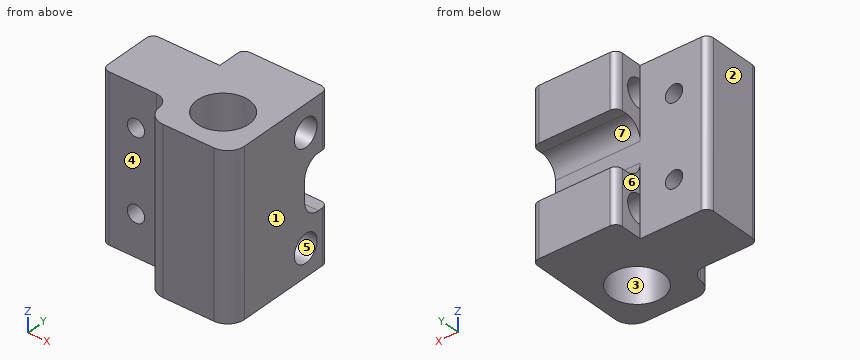
from build123d import *

# Parameters (mm, degrees)
SKETCH_1_W          = 25
SKETCH_1_H          = 48
EXTRUDE_1_DEPTH     = 25
SKETCH_2_R          = 7.65
CUT_EXTRUDE_1_DEPTH = 57.57461336
SKETCH_3_W          = 25
SKETCH_3_H          = 48
EXTRUDE_2_DEPTH     = 10
SKETCH_4_R          = 4.1
CUT_EXTRUDE_2_DEPTH = 53.240311871
FILLET_1_R          = 5
SKETCH_6_W          = 48
SKETCH_6_H          = 18
EXTRUDE_3_DEPTH     = 20
SKETCH_7_R          = 2.55
CUT_EXTRUDE_3_DEPTH = 54.919821703
FILLET_3_R          = 4
SKETCH_8_W          = 25
SKETCH_8_H          = 16
CUT_EXTRUDE_4_DEPTH = 8.406306785
FILLET_4_R          = 5
FILLET_5_R          = 2
FILLET_6_R          = 2


with BuildPart() as part:
    # 草图1 → 凸台-拉伸1 (new body)
    with BuildSketch(Plane(origin=(0, 0, 0), x_dir=(1, 0, 0), z_dir=(0, 1, 0))):
        with Locations((-3.982926829, 5.648780488)):
            Rectangle(SKETCH_1_W, SKETCH_1_H)
    extrude(amount=EXTRUDE_1_DEPTH)

    # 草图2 → 切除-拉伸1 (cut, through all)
    with BuildSketch(Plane.XY.offset(18.351219512)):
        with Locations((-3.982926829, 12.5)):
            Circle(SKETCH_2_R)
    extrude(amount=-CUT_EXTRUDE_1_DEPTH, mode=Mode.SUBTRACT)

    # 草图3 → 凸台-拉伸2 (add)
    with BuildSketch(Plane(origin=(0, 25, 0), x_dir=(1, 0, 0), z_dir=(0, 1, 0))):
        with Locations((-3.982926829, 5.648780488)):
            Rectangle(SKETCH_3_W, SKETCH_3_H)
    extrude(amount=EXTRUDE_2_DEPTH)

    # 草图4 → 切除-拉伸2 (cut, through all)
    with BuildSketch(Plane(origin=(8.517073171, 0, 0), x_dir=(0, 0, -1), z_dir=(1, 0, 0))):
        with Locations((-10.351219512, 27)):
            Circle(SKETCH_4_R)
        with Locations((21.648780488, 27)):
            Circle(SKETCH_4_R)
    extrude(amount=-CUT_EXTRUDE_2_DEPTH, mode=Mode.SUBTRACT)

    # 圆角1
    fillet_1_edges = [part.edges().sort_by_distance(p)[0] for p in [
        (8.517073171, 0, -5.648780488),
        (-16.482926829, 0, -5.648780488),
    ]]
    fillet(fillet_1_edges, radius=FILLET_1_R)

    # 草图6 → 凸台-拉伸3 (add)
    with BuildSketch(Plane.ZY.offset(16.482926829)):
        with Locations((-5.648780488, 17.593693215)):
            Rectangle(SKETCH_6_W, SKETCH_6_H)
    extrude(amount=EXTRUDE_3_DEPTH)

    # 草图7 → 切除-拉伸3 (cut, through all)
    with BuildSketch(Plane.XZ.offset(-8.593693215)):
        with Locations(Location((-26.482926829, 6.251219512, 0), (0, 0, 270))):
            Circle(SKETCH_7_R)
        with Locations(Location((-26.482926829, -17.548780488, 0), (0, 0, 270))):
            Circle(SKETCH_7_R)
    extrude(amount=-CUT_EXTRUDE_3_DEPTH, mode=Mode.SUBTRACT)

    # 圆角3
    fillet_3_edges = [part.edges().sort_by_distance(p)[0] for p in [
        (-16.482926829, 8.593693215, -5.648780488),
    ]]
    fillet(fillet_3_edges, radius=FILLET_3_R)

    # 草图8 → 切除-拉伸4 (cut)
    with BuildSketch(Plane(origin=(0, 35, 0), x_dir=(1, 0, 0), z_dir=(0, 1, 0))):
        with Locations((-3.982926829, 5.648780488)):
            Rectangle(SKETCH_8_W, SKETCH_8_H)
    extrude(amount=-CUT_EXTRUDE_4_DEPTH, mode=Mode.SUBTRACT)

    # 圆角4
    fillet_4_edges = [part.edges().sort_by_distance(p)[0] for p in [
        (-3.982926829, 26.593693215, 2.351219512),
        (-3.982926829, 26.593693215, -13.648780488),
    ]]
    fillet(fillet_4_edges, radius=FILLET_4_R)

    # 圆角5
    fillet_5_edges = [part.edges().sort_by_distance(p)[0] for p in [
        (-36.482926829, 26.593693215, -5.648780488),
        (-36.482926829, 8.593693215, -5.648780488),
    ]]
    fillet(fillet_5_edges, radius=FILLET_5_R)

    # 圆角6
    fillet_6_edges = [part.edges().sort_by_distance(p)[0] for p in [
        (-16.482926829, 35, -21.648780488),
        (8.517073171, 35, 10.351219512),
        (-16.482926829, 35, 10.351219512),
        (8.517073171, 35, -21.648780488),
    ]]
    fillet(fillet_6_edges, radius=FILLET_6_R)


solid = part.part
Source: CAD feature listing. Evaluate the final solid. Frame: model axes, mm. Face numbers are marked on the shaded views. A direction names the side the tool comes from. Give positions to 0.01 mm unless a question says otherwise; leave off trailing zeros. Write each loop counter-clockwise with the first axis right and the second up, starting at its lowest first coordinate (ties: lowest second). Pieces come first, ordered by that corner, then holes. Notation, with made-up numbers: M 15,-7 L 53,-7 A17 cw 53,18 Z; hole C -25.5,-13 d1. An arc over 180 degrees is marked long. Return JSON: item names as keys, results as strings. Group by question number.
1) Cut plane D-D, the plane z = -21. Give the number of separate pieces and of enclosed holes in the cut face, then the cut area to 3 significant figures.
2) First-contact query: pin 1 Ø10 at (x, z) = (-23.5, 4.5) entering from +Y; pin 2 Ø5 at (y, z) = (30, 9) entering from -X; pin 3 Ø5 at (y, z) = (27, -21.65) entering from +X. Flat tips, straight axial feed; report the tip coordinate or a pass-through.
3) Set-up query: the marked faces 4, 5, 6 and 7. Return all of +Z, -Z, +X, -X, +Y, -Y with unobstructed straight access to the full face (end or side cutting, diameter ignored); none if empty.
4) Draft query along X for the marked faces 1, 2 and 3. Return one class per face: released by +X, released by -X, zero draft, split by the parting line, or undercut.
5) Cut plane B-B, the plane y = 28. Output: boundary loops of the cut face in (x, z), then the cut area to 3 significant figures.
6) Cut plane A-A, the plane x = -5.5. Output: boundary loops of the cut face in (y, z), then the cut area to 3 significant figures.
7) Ray query, L1, parallel to Z at x = -26.5, y = 17; L2, parallel to Z at x = -25.5, y = 24; L3, parallel to Y at x = -3, z = 10. Return the intervals inside material, ascending.
8) Cut plane C-C, the plane y = 12.5. Output: boundary loops of the cut face in (x, z).
Data:
{
 "1": {"separate pieces": "2", "enclosed holes": "1", "area": "838 mm²"},
 "2": {"pin 1": "stops at y = 26.59", "pin 2": "stops at x = -16.48", "pin 3": "stops at x = -16.48"},
 "3": {"face 4": "+Z, -Z, -X, -Y", "face 5": "+X", "face 6": "+Z, -Z, -X, +Y", "face 7": "+X, -X, +Y"},
 "4": {"face 1": "released by +X", "face 2": "released by -X", "face 3": "undercut"},
 "5": {"outline": "M -16.48,-29.65 L 8.52,-29.65 L 8.52,-25.62 L -16.48,-25.62 Z; M -16.48,-17.67 L 8.52,-17.67 L 8.52,-12.13 L -16.48,-12.13 Z; M -16.48,0.83 L 8.52,0.83 L 8.52,6.38 L -16.48,6.38 Z; M -16.48,14.33 L 8.52,14.33 L 8.52,18.35 L -16.48,18.35 Z", "area": "479 mm²"},
 "6": {"outline": "M 0,-29.65 L 5,-29.65 L 5,18.35 L 0,18.35 Z; M 20,-29.65 L 35,-29.65 L 35,-13.65 L 31.59,-13.65 A5 cw 26.59,-8.65 L 26.59,-2.65 A5 cw 31.59,2.35 L 35,2.35 L 35,18.35 L 20,18.35 Z; hole C 27,-21.65 d8.2; hole C 27,10.35 d8.2", "area": "731 mm²"},
 "7": {"L1": "z = -29.65 to -20.1, -15 to 3.7, 8.8 to 18.35", "L2": "z = -29.65 to -19.9, -15.2 to 3.9, 8.6 to 18.35", "L3": "y = 0 to 4.91, 20.09 to 22.92, 31.08 to 35"},
 "8": {"outline": "M -36.48,-29.65 L -11.63,-29.65 L -11.63,18.35 L -36.48,18.35 Z; M 3.67,-29.65 L 8.52,-29.65 L 8.52,18.35 L 3.67,18.35 Z; hole C -26.48,-17.55 d5.1; hole C -26.48,6.25 d5.1"}
}
